Geometry check sheet. Reference: drawing and pictorial views, mm from the part's lowest x, y, z. A direction names the side the tool comes from. Coordinates: 2 decimals unless noted, no trailing zeros. Loops run counter-clockwise (first coordinate to the right, second up) from the corner with the lowest first, then second, coordinate; pieces in that order, holes last. Notation, with made-up numbers: (71, 59) -> (83, 59) arc R27 ccw to (83, 95) -> close; hole circle Ø11 at (1, 81). An arc over 180 degrees is marked (long way). Use CSV: the item, a comma, the result in double quotes.
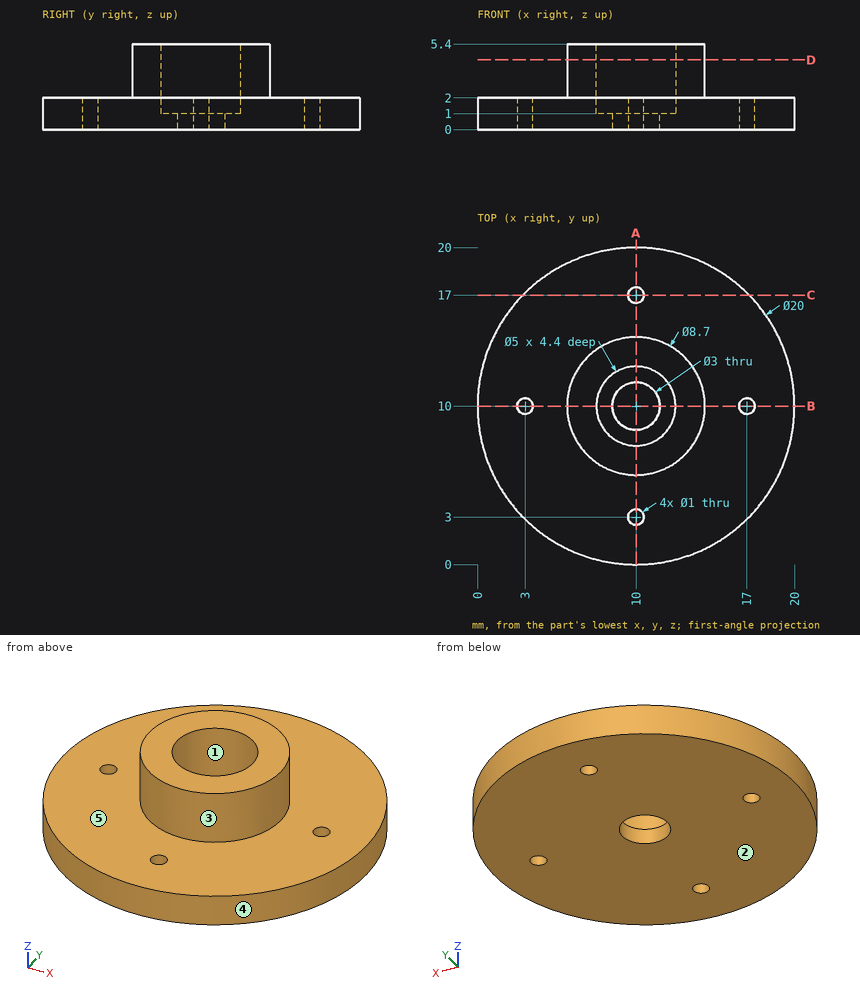
1) Cross-section at A-A on x = 10. Record the boundary of the cut face in (y, z).
Answer below:
outline,"(0, 0) -> (2.5, 0) -> (2.5, 2) -> (0, 2) -> close; (3.5, 0) -> (8.5, 0) -> (8.5, 1) -> (7.5, 1) -> (7.5, 5.4) -> (5.65, 5.4) -> (5.65, 2) -> (3.5, 2) -> close; (11.5, 0) -> (16.5, 0) -> (16.5, 2) -> (14.35, 2) -> (14.35, 5.4) -> (12.5, 5.4) -> (12.5, 1) -> (11.5, 1) -> close; (17.5, 0) -> (20, 0) -> (20, 2) -> (17.5, 2) -> close"
2) Cross-section at D-D on z = 4.4. Record the boundary of the cut face in (x, y), and give its area (3 significant figures).
Answer below:
outline,"circle Ø8.7 at (10, 10); hole circle Ø5 at (10, 10)"
area,"39.8 mm²"
3) Go/stop test with flat-tipped pins: pin 1 Ø4 at (x, y) = (10, 10) entering from +Z; pin 2 Ø3 at (x, z) = (14, 4.5) entering from -Y; pin 3 Ø1 at (y, z) = (11.5, 1) entering from -X. Record where each tip stops, or that it passes through.
Answer below:
pin 1,"stops at z = 1"
pin 2,"stops at y = 6.44"
pin 3,"stops at x = 0.05"
4) Thickness scan on line 1 along Y through (x, z) = (10, 0.45); line 2 along X through (y, z) = (17, 0.7); line 3 along Z through (x, y) = (11.5, 4). Record the ranges inside material, lowest first. Write a range as from..to.
Answer below:
line 1,"y = 0..2.5, 3.5..8.5, 11.5..16.5, 17.5..20"
line 2,"x = 2.86..9.5, 10.5..17.14"
line 3,"z = 0..2"
5) Cross-section at C-C on y = 17. Record the boundary of the cut face in (x, z), and give its area (3 significant figures).
Answer below:
outline,"(2.86, 0) -> (9.5, 0) -> (9.5, 2) -> (2.86, 2) -> close; (10.5, 0) -> (17.14, 0) -> (17.14, 2) -> (10.5, 2) -> close"
area,"26.6 mm²"
6) Access from +Z, -Z, +X, -X, +Y, -Y to the whole of each face (thin tool, end or side, straight path). Record for the marked faces 4 and 5.
Answer below:
face 4,"+Z, -Z"
face 5,"+Z"
7) Draft check along Y on the marked faces 1, 2 and 3. Enter one of: released by +Y, released by -Y, zero draft, split by the parting line, or undercut.
Answer below:
face 1,"undercut"
face 2,"zero draft"
face 3,"split by the parting line"
